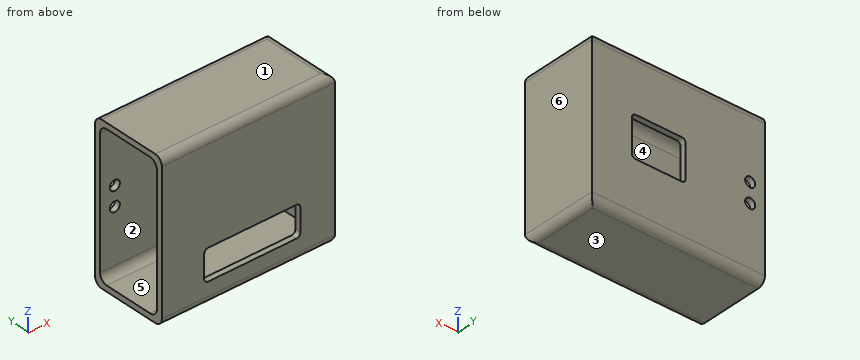
```python
from build123d import *

# Parameters (mm, degrees)
SKETCH1_W           = 50.8
SKETCH1_H           = 25.4
BOSS_EXTRUDE1_DEPTH = 57.15
SHELL1_T            = -1.905
SKETCH2_W           = 17.78
SKETCH2_H           = 13.335
CUT_EXTRUDE1_DEPTH  = 12.7
SKETCH3_W           = 31.75
SKETCH3_H           = 10.16
CUT_EXTRUDE2_DEPTH  = 12.7
FILLET1_R           = 2.54
FILLET2_R           = 1.27
FILLET3_R           = 1.27
SKETCH5_R           = 1.651
CUT_EXTRUDE3_DEPTH  = 2.54


with BuildPart() as part:
    # Sketch1 → Boss-Extrude1 (new body)
    with BuildSketch(Plane(origin=(0, 0, 0), x_dir=(0, 0, -1), z_dir=(1, 0, 0))):
        Rectangle(SKETCH1_W, SKETCH1_H)
    extrude(amount=BOSS_EXTRUDE1_DEPTH)

    # Shell1
    shell1_openings = [part.faces().sort_by_distance(p)[0] for p in [
        (0, 0, 0),
    ]]
    offset(amount=SHELL1_T, openings=shell1_openings, kind=Kind.INTERSECTION)

    # Sketch2 → Cut-Extrude1 (cut)
    with BuildSketch(Plane(origin=(0, 12.7, 0), x_dir=(1, 0, 0), z_dir=(0, 1, 0))):
        with Locations((35.0974914, 0)):
            Rectangle(SKETCH2_W, SKETCH2_H)
    extrude(amount=-CUT_EXTRUDE1_DEPTH, mode=Mode.SUBTRACT)

    # Sketch3 → Cut-Extrude2 (cut)
    with BuildSketch(Plane.XZ.offset(12.7)):
        with Locations((29.845, -13.335)):
            Rectangle(SKETCH3_W, SKETCH3_H)
    extrude(amount=-CUT_EXTRUDE2_DEPTH, mode=Mode.SUBTRACT)

    # Fillet1
    fillet1_edges = [part.edges().sort_by_distance(p)[0] for p in [
        (57.15, 0, 25.4),
        (27.6225, -10.795, -23.495),
        (27.6225, 10.795, -23.495),
        (27.6225, 10.795, 23.495),
        (27.6225, -10.795, 23.495),
        (57.15, 0, -25.4),
        (28.575, -12.7, -25.4),
        (28.575, -12.7, 25.4),
        (28.575, 12.7, 25.4),
        (28.575, 12.7, -25.4),
    ]]
    fillet(fillet1_edges, radius=FILLET1_R)

    # Fillet2
    fillet2_edges = [part.edges().sort_by_distance(p)[0] for p in [
        (26.2074914, 11.7475, 6.6675),
        (26.2074914, 11.7475, -6.6675),
        (43.9874914, 11.7475, -6.6675),
        (43.9874914, 11.7475, 6.6675),
    ]]
    fillet(fillet2_edges, radius=FILLET2_R)

    # Fillet3
    fillet3_edges = [part.edges().sort_by_distance(p)[0] for p in [
        (45.72, -11.7475, -8.255),
        (45.72, -11.7475, -18.415),
        (13.97, -11.7475, -18.415),
        (13.97, -11.7475, -8.255),
    ]]
    fillet(fillet3_edges, radius=FILLET3_R)

    # Sketch5 → Cut-Extrude3 (cut)
    with BuildSketch(Plane(origin=(0, 12.7, 0), x_dir=(1, 0, 0), z_dir=(0, 1, 0))):
        with Locations(Location((4.8875, 3.243405994, 0), (0, 0, 270))):
            Circle(SKETCH5_R)
        with Locations(Location((4.8875, -3.156594006, 0), (0, 0, 270))):
            Circle(SKETCH5_R)
    extrude(amount=-CUT_EXTRUDE3_DEPTH, mode=Mode.SUBTRACT)


solid = part.part
```
Work out the finished part from the listing and answer in its coordinate system (mm). Face numbers are marked on the shaded views. A direction names the side the tool comes from. Round coordinates to 2 decimals unless told otherwise and drop trailing zeros. Write each loop counter-clockwise with the first axis right and the second up, starting at its lowest first coordinate (ties: lowest second). Pieces come first, ordered by that corner, then holes.
1) Which of the six approach directions +Z, -Z, +X, -X, +Y, -Y give full straight-line access (tool end or side, diameter ignored) to the marked faces 1 and 2?
2) A cutting plane is placed at A-A on x = 35.5. Determine the outline of the cut face in (y, z) (1 decimal), and give its area (3 significant figures).
3) Determine the mould class of the marked faces 3, 4, 5 and 6 for opening direction Z: pulls with the +Z half, pulls with the -Z half, needs draft (parallel to the pull), parting line crosses it, or undercut.
4) Consider probe 1 along Y at (x, z) = (17, 15) (3 decimals); probe 2 along Z at (x, y) = (23, 5.75) (3 decimals); probe 3 along X at (y, z) = (-11, -12). Determine where each line is inside the solid, lowest interval first.
5) Flat-ended cylindrical pins translate along their axes: P1, Ø12, axis at y = -2, z = 5, coming from the -X side (3 decimals); P2, Ø2, axis at x = 4.89, z = -3.24, coming from the +Y side (3 decimals); P3, Ø0.6, axis at x = 29, y = -12, coming from the -Z side. Find the tip coordinate at first contact, or state that the pin passes through.
6) A cutting plane is placed at D-D on y = -2. Determine the outline of the cut face in (x, z) (3 decimals).
7) A cutting plane is placed at C-C on z = -4. Give the number of separate pieces and of enclosed holes in the cut face, and give its area (3 significant figures).
8) A cutting plane is placed at B-B on z = -15. Determine the outline of the cut face in (x, y) (3 decimals).
Entries:
1. face 1: +Z, +X, -X, +Y, -Y
1. face 2: -X
2. outline: (-12.7, -22.9) arc R2.5 ccw to (-10.2, -25.4) - (10.2, -25.4) arc R2.5 ccw to (12.7, -22.9) - (12.7, -6.7) - (10.8, -6.7) - (10.8, -21) arc R2.5 cw to (8.3, -23.5) - (-8.3, -23.5) arc R2.5 cw to (-10.8, -21) - (-10.8, -18.4) - (-12.7, -18.4) - close; (-12.7, -8.3) - (-10.8, -8.3) - (-10.8, 21) arc R2.5 cw to (-8.3, 23.5) - (8.3, 23.5) arc R2.5 cw to (10.8, 21) - (10.8, 6.7) - (12.7, 6.7) - (12.7, 22.9) arc R2.5 ccw to (10.2, 25.4) - (-10.2, 25.4) arc R2.5 ccw to (-12.7, 22.9) - close
2. area: 231 mm2
3. face 3: pulls with the -Z half
3. face 4: undercut
3. face 5: undercut
3. face 6: needs draft
4. probe 1: y = -12.7 to -10.795, 10.795 to 12.7
4. probe 2: z = -25.4 to -23.495, 23.495 to 25.4
4. probe 3: x = 0 to 13.97, 45.72 to 57.15
5. P1: stops at x = 55.245
5. P2: stops at y = -10.795
5. P3: stops at z = -24.88
6. outline: (0, -25.4) - (54.61, -25.4) arc R2.54 ccw to (57.15, -22.86) - (57.15, 22.86) arc R2.54 ccw to (54.61, 25.4) - (0, 25.4) - (0, 23.495) - (55.245, 23.495) - (55.245, -23.495) - (0, -23.495) - close
7. separate pieces: 3
7. enclosed holes: 0
7. area: 219 mm2
8. outline: (0, -12.7) - (13.97, -12.7) - (13.97, -10.795) - (0, -10.795) - close; (0, 10.795) - (55.245, 10.795) - (55.245, -10.795) - (45.72, -10.795) - (45.72, -12.7) - (57.15, -12.7) - (57.15, 12.7) - (0, 12.7) - close
